Read the model definition and answer for the solid it produces. Units are mm, in the model's axes. Give positions to 0.01 mm unless a question says otherwise; leave off trailing zeros. Write each loop counter-clockwise with the first axis right and the second up, starting at its lowest first coordinate (ties: lowest second). Pieces come first, ordered by that corner, then holes. Notation, with made-up numbers: M 52,83.5 L 75,83.5 A16 cw 75,98.5 Z; hole C 66,54 d4. An arc over 180 degrees is marked long. Use a Markdown table: item, result. Add a question column.
Item 1: A cutting plane is placed at A-A on x = 54.5. Determine the outline of the cut face in (y, z), then the cut area to 4 significant figures.
Item 2: Consider probe 1 along Z at (x, y) = (54.5, 5.5); probe 2 along X at (y, z) = (6.55, 11); probe 3 along Z at (x, y) = (55.5, 5.6). Determine where each line is inside the solid, lowest interval first. Write a range as [from, to].
Item 3: A cutting plane is placed at B-B on z = 34.8. Determine the outline of the cut face in (x, y).
Item 4: A cutting plane is placed at C-C on y = 5.7. Determine the outline of the cut face in (x, z).
Item 5: The mould has two halves that part along X. Classify faces 1 (the cylindrical face through (55.306, 5.838, 33.535)), 2 (the flat face through (58, 6, 22)), 3 (the cylindrical face through (2.305, 5.838, 33.313)), 4 (the flat face through (29, 6, 6)): pulls with the +X half, pulls with the -X half, needs draft (parallel to the pull), parting line crosses it, or undercut.
from build123d import *

# Parameters (mm, degrees)
CYLINDER_R       = 1.5
CYLINDER_DEPTH   = 10
ARRAY001_X_COUNT = 2
ARRAY001_X_PITCH = 52
ARRAY001_Z_COUNT = 2
ARRAY001_Z_PITCH = 25
BOX002_W         = 58
BOX002_H         = 1.7
BOX002_DEPTH     = 31.5


with BuildPart() as hole_array_clone:
    # Cylinder → Cylinder (new body)
    with BuildSketch(Plane(origin=(0, 0, 0), x_dir=(1, 0, 0), z_dir=(0, 1, 0))):
        Circle(CYLINDER_R)
    extrude(amount=CYLINDER_DEPTH)

    # Array001 X: hole array clone ×2


with BuildPart() as hole_array_clone_1:
    add(hole_array_clone.part)
    with Locations(*[(i * ARRAY001_X_PITCH, 0, 0) for i in range(1, ARRAY001_X_COUNT)]):
        add(hole_array_clone.part)

    # Array001 Z: hole array clone ×2


with BuildPart() as hole_array_clone_2:
    add(hole_array_clone_1.part)
    with Locations(*[(0, 0, i * ARRAY001_Z_PITCH) for i in range(1, ARRAY001_Z_COUNT)]):
        add(hole_array_clone_1.part)


with BuildPart() as hole_array_clone_3:
    # Array001 placement: moved
    add(hole_array_clone_2.part.moved(Location((3, 0, 9.25))))


with BuildPart() as hole_array_clone_4:
    # Clone001 placement: moved
    add(hole_array_clone_3.part.moved(Location((-0.5, 0, 0.55))))


with BuildPart() as pcb_mockup:
    # Box002 → Box002 (new body)
    with BuildSketch(Plane(origin=(0, 5, 6), x_dir=(1, 0, 0), z_dir=(0, 0, 1))):
        with Locations((29, 0.85)):
            Rectangle(BOX002_W, BOX002_H)
    extrude(amount=BOX002_DEPTH)

    # Cut: cut hole array clone
    add(hole_array_clone_4.part, mode=Mode.SUBTRACT)


solid = pcb_mockup.part
Filled in:
| question | item | result |
|---|---|---|
| 1 | outline | M 5,6 L 6.7,6 L 6.7,8.3 L 5,8.3 Z; M 5,11.3 L 6.7,11.3 L 6.7,33.3 L 5,33.3 Z; M 5,36.3 L 6.7,36.3 L 6.7,37.5 L 5,37.5 Z |
| 1 | area | 43.35 mm² |
| 2 | probe 1 | [6, 8.3], [11.3, 33.3], [36.3, 37.5] |
| 2 | probe 2 | [0, 1.6], [3.4, 53.6], [55.4, 58] |
| 2 | probe 3 | [6, 8.68], [10.92, 33.68], [35.92, 37.5] |
| 3 | outline | M 0,5 L 1,5 L 1,6.7 L 0,6.7 Z; M 4,5 L 53,5 L 53,6.7 L 4,6.7 Z; M 56,5 L 58,5 L 58,6.7 L 56,6.7 Z |
| 4 | outline | M 0,6 L 58,6 L 58,37.5 L 0,37.5 Z; hole C 2.5,9.8 d3; hole C 2.5,34.8 d3; hole C 54.5,9.8 d3; hole C 54.5,34.8 d3 |
| 5 | face 1 | undercut |
| 5 | face 2 | pulls with the +X half |
| 5 | face 3 | undercut |
| 5 | face 4 | needs draft |
